Build history of the part. All positions in model axes, mm. Face numbers are marked on the shaded views. A direction names the side the tool comes from. Give positions to 0.01 mm unless a question says otherwise; leave off trailing zeros. Write each loop counter-clockwise with the first axis right and the second up, starting at its lowest first coordinate (ties: lowest second). Pieces come first, ordered by that corner, then holes. Notation, with made-up numbers: (9, 0.25) -> (28, 0.25) arc R23 ccw to (28, 18.25) -> close; hole circle Ø7 at (-2, -1.75). An arc over 180 degrees is marked (long way). One line per question, with ' | ' between items. Start each with the question number.
(1) Drill centre lines: probe 1 along X at (y, z) = (7.75, 63.5); probe 2 along X at (y, z) = (9.75, -38.1); probe 3 along Z at (x, y) = (37, 3.5). Where is each one in solid material? Low to high. Write a range as from..to.
(2) Band-saw the part on D-D, the plane z = 38.1. Give the cut face in (x, y).
(3) Band-saw the part on A-A, the plane x = 0. Give the cut face in (y, z) (3 decimals), and give its area (3 significant figures).
(4) Band-saw the part on B-B, the plane x = -76.2. Give the cut face in (y, z), and give its area (3 significant figures).
(5) Band-saw the part on C-C, the plane x = -38.1. Give the cut face in (y, z), and give its area (3 significant figures).
(6) Tool access for the marked faces 1 and 2: list every direction of +Z, -Z, +X, -X, +Y, -Y with a clear straight run to the whole face (end or side of a thin tool).
(7) Pull direction X, two halves, no side cores. Call the marked faces 3, 4 and 5: released by +X, released by -X, zero draft, split by the parting line, or undercut.
(8) Pin check, flat tips, straight feed: P1, Ø5, axis at x = 76.2, z = 0, coming from the +Y side; P2, Ø6, axis at y = 8, z = 59.5, coming from the -X side; P3, Ø1.5, axis at x = -35.5, y = 2, coming from the -Z side; P4, Ø3, axis at x = -53.5, y = 4.5, coming from the +Z side. Stop position of each tip, or through.
from build123d import *

# Parameters (mm, degrees)
SKETCH2_W                = 88.9
SKETCH2_H                = 12.7
CUT_EXTRUDE1_DEPTH       = 13.7
F_5_16_CLEARANCE_HOLE1_D = 8.4328
CIRPATTERN1_COUNT        = 12
F_5_16_CLEARANCE_HOLE2_D = 10.16


with BuildPart() as part:
    # Sketch2 → Revolve1 (revolve)
    with BuildSketch(Plane.XY):
        with Locations((-44.45, 6.35)):
            Rectangle(SKETCH2_W, SKETCH2_H)
    revolve(axis=Axis((0, 12.7, 0), (0, -1, 0)))

    # Sketch3 → Cut-Extrude1 (cut, through all)
    with BuildSketch(Plane(origin=(0, 12.7, 0), x_dir=(1, 0, 0), z_dir=(0, 1, 0))):
        with BuildLine():
            Line((-12.7, 34.925), (-12.7, -34.925))
            ThreePointArc((-12.7, -34.925), (0, -47.625), (12.7, -34.925))
            Line((12.7, -34.925), (12.7, 34.925))
            ThreePointArc((12.7, 34.925), (0, 47.625), (-12.7, 34.925))
        make_face()
    extrude(amount=-CUT_EXTRUDE1_DEPTH, mode=Mode.SUBTRACT)

    # 5_16 Clearance Hole1 (through all)
    with Locations(Plane(origin=(0, 12.7, 0), x_dir=(1, 0, 0), z_dir=(0, 1, 0))):
        with Locations((0, 76.2)):
            f_5_16_clearance_hole1 = Hole(F_5_16_CLEARANCE_HOLE1_D / 2)

    # CirPattern1: 5_16 Clearance Hole1 ×12 about axis
    cirpattern1_axis = Axis((0, 0, 0), (0, 1, 0))
    for i in range(1, CIRPATTERN1_COUNT):
        add(f_5_16_clearance_hole1.rotate(cirpattern1_axis, i * 360 / CIRPATTERN1_COUNT), mode=Mode.SUBTRACT)

    # 5_16 Clearance Hole2 (through all)
    with Locations(Plane(origin=(0, 12.7, 0), x_dir=(1, 0, 0), z_dir=(0, 1, 0))):
        with Locations((31.75, 0)):
            Hole(F_5_16_CLEARANCE_HOLE2_D / 2)


solid = part.part
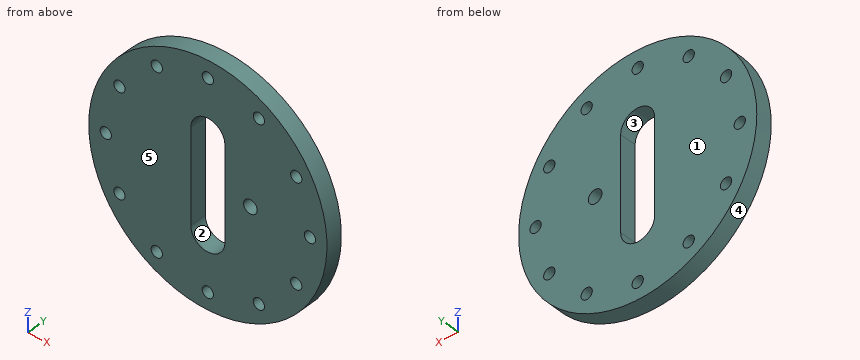
Results:
1) probe 1: x = -62.22..-41.5, -34.7..34.7, 41.5..62.22 | probe 2: x = -80.32..-70.21, -61.77..-12.3, 12.3..61.77, 70.21..80.32 | probe 3: z = -80.83..-70.06, -61.92..61.92, 70.06..80.83
2) outline: (-80.32, 0) -> (-70.21, 0) -> (-70.21, 12.7) -> (-80.32, 12.7) -> close; (-61.77, 0) -> (-12.3, 0) -> (-12.3, 12.7) -> (-61.77, 12.7) -> close; (12.3, 0) -> (61.77, 0) -> (61.77, 12.7) -> (12.3, 12.7) -> close; (70.21, 0) -> (80.32, 0) -> (80.32, 12.7) -> (70.21, 12.7) -> close
3) outline: (0, -88.9) -> (12.7, -88.9) -> (12.7, -80.416) -> (0, -80.416) -> close; (0, -71.984) -> (12.7, -71.984) -> (12.7, -47.625) -> (0, -47.625) -> close; (0, 47.625) -> (12.7, 47.625) -> (12.7, 71.984) -> (0, 71.984) -> close; (0, 80.416) -> (12.7, 80.416) -> (12.7, 88.9) -> (0, 88.9) -> close | area: 834 mm²
4) outline: (0, -45.79) -> (12.7, -45.79) -> (12.7, -4.22) -> (0, -4.22) -> close; (0, 4.22) -> (12.7, 4.22) -> (12.7, 45.79) -> (0, 45.79) -> close | area: 1,060 mm²
5) outline: (0, -80.32) -> (12.7, -80.32) -> (12.7, -70.21) -> (0, -70.21) -> close; (0, -61.77) -> (12.7, -61.77) -> (12.7, 61.77) -> (0, 61.77) -> close; (0, 70.21) -> (12.7, 70.21) -> (12.7, 80.32) -> (0, 80.32) -> close | area: 1,830 mm²
6) face 1: +Z, -Z, +X, -X, +Y | face 2: +Y, -Y
7) face 3: undercut | face 4: split by the parting line | face 5: zero draft
8) P1: passes through | P2: stops at x = -68.64 | P3: stops at z = -81.83 | P4: stops at z = 72.11
